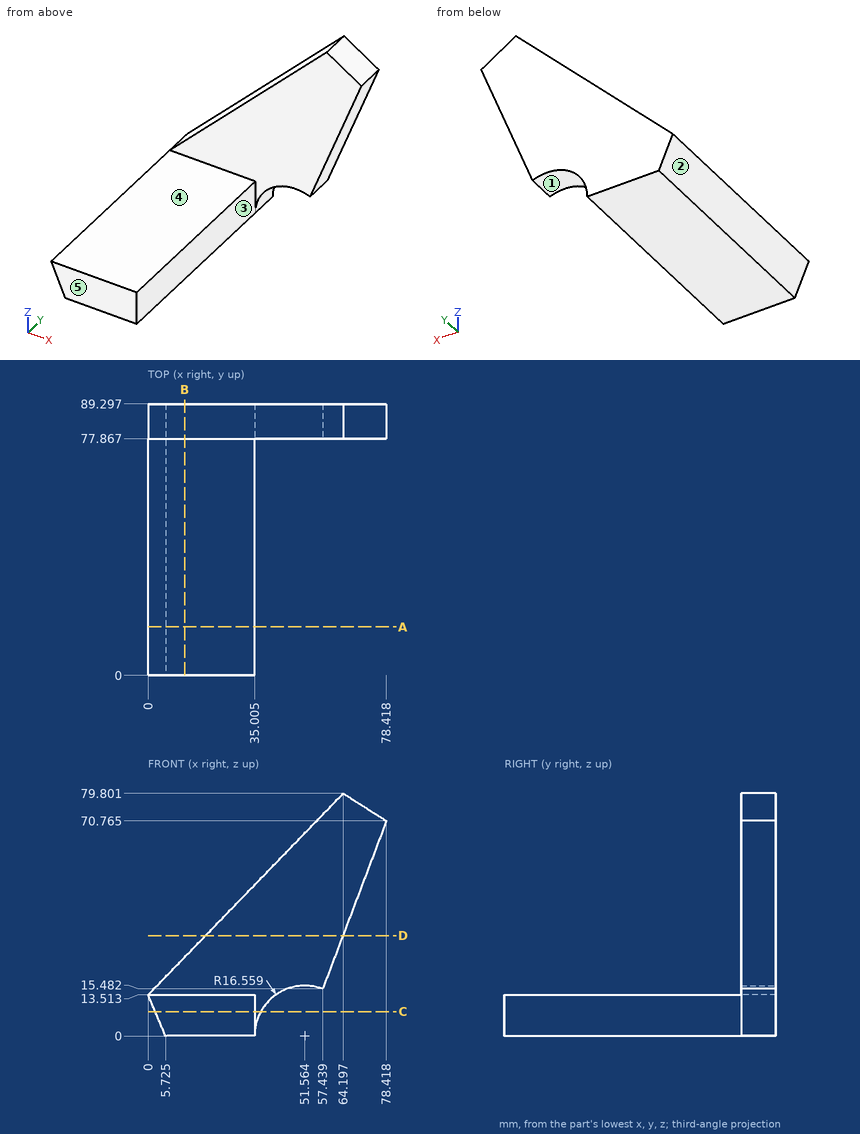
Geometry: see drawing. Coordinates: mm, zero at the bounding-box minimum. A direction names the side the tool comes from. Coordinates: 2 decimals unless noted, no trailing zeros. Write each loop counter-clockwise with the first axis right and the second up, starting at its lowest first coordinate (ties: lowest second). Pieces come first, ordered by that corner, then holes. Notation, with made-up numbers: M 51.25,-26 L 95.25,-26 A26 ccw 95.25,1 Z; hole C 58.5,-23 d6. An arc over 180 degrees is marked long. Use CSV: the item, a comma, the result in double quotes. Start each with the question number.
1. Cut plane D-D on z = 33. Return the cut outline in (x, y).
2. Cut plane B-B on x = 12. Return the cut outline in (y, z) (1 decimal), plus the area to 3 significant figures.
3. Cut plane A-A on y = 16. Return the cut outline in (x, z) (1 decimal).
4. Cut plane C-C on z = 8. Return the cut outline in (x, y) (1 decimal).
5. Reachability of the marked faces 4 and 5 from +Z, -Z, +X, -X, +Y, -Y: full face, straight path, thin tool, end or side. Return the list, or none.
6. Mould query, pull axis X, two halves, no side actions, for the marked faces 1, 2 and 3. Classes: pulls with the +X half, pulls with the -X half, needs draft (parallel to the pull), parting line crosses it, or undercut.
7. First-contact query: P1, Ø3, axis at x = 23.5, y = 20.5, coming from the +Z side; P2, Ø4, axis at y = 48, z = 3.5, coming from the +X side (1 decimal); P3, Ø5, axis at x = 51, y = 75.5, coming from the -Z side; P4, Ø12, axis at y = 68, z = 67.5, coming from the -X side. Flat tips, straight axial feed; report the tip coordinate or a pass-through.
8. Ray query, probe 1 along Y at (x, z) = (59.5, 44.5); probe 2 along Z at (x, y) = (25, 44); probe 3 along X at (y, z) = (69.5, 5) (1 decimal). Return the intervals inside material, ascending.
Entries:
1,outline,"M 18.87,77.87 L 64.09,77.87 L 64.09,89.3 L 18.87,89.3 Z"
2,outline,"M 0,0 L 89.3,0 L 89.3,25.9 L 77.9,25.9 L 77.9,13.5 L 0,13.5 Z"
2,area,"1,350 mm²"
3,outline,"M 0,13.5 L 5.7,0 L 35,0 L 35,13.5 Z"
4,outline,"M 2.3,0 L 35,0 L 35,77.9 L 37.1,77.9 L 37.1,89.3 L 2.3,89.3 Z"
5,face 4,"+Z, +X, -X, -Y"
5,face 5,"+Z, -Z, +X, -X, -Y"
6,face 1,"undercut"
6,face 2,"pulls with the -X half"
6,face 3,"pulls with the +X half"
7,P1,"z = 13.51"
7,P2,"x = 35"
7,P3,"z = 16.5"
7,P4,"through"
8,probe 1,"77.87 to 89.3"
8,probe 2,"0 to 13.51"
8,probe 3,"3.6 to 35"
